Could you check a few things on this model? Use its own coordinates, in mm. A direction names the side the tool comes from. Round coordinates to 2 decimals unless told otherwise and drop trailing zeros. Loops run counter-clockwise (first coordinate to the right, second up) from the corner with the lowest first, then second, coordinate; pieces in that order, holes last. Notation, with made-up numbers: (15, 14.5) -> (31, 14.5) arc R22 ccw to (31, 52.5) -> close; hole circle Ø2 at (78.25, 31). An arc over 180 degrees is marked (long way). Write each question's results on one line, items separated by ' | '. Start each with the question number.
1) Imagine slicing it at B-B, the plane x = 0. List the corners of the cut face in (y, z) for me.
2) We'd pull the mould along X, two halves only. Please class faces 4 (the cylindrical face through (9.886, 0.74, 10.078)), 5 (the cylindrical face through (-0.108, 2.486, 0.488)), 6 (the flat face through (0, 0, 0)): pulls with the +X half, pulls with the -X half, needs draft (parallel to the pull), parting line crosses it, or undercut.
3) Imagine slicing it at C-C, the plane z = 2.5. List the corners of the cut face in (x, y) for me.
4) If I drill on probe 1 along Y at (x, z) = (9.5, -1.75); probe 2 along X at (y, z) = (1.2, -4); probe 3 along Y at (x, z) = (-4, 11.5), over which ranges is the centre line in solid material (lowest first)?
5) For P1, Ø1.3, axis at y = 3, z = 12.5, coming from the -X side; P2, Ø1.3, axis at y = 3, z = -13.5, coming from the +X side; P3, Ø1, axis at y = 4.5, z = -3, coming from the +X side; P4, Ø0.8, axis at x = 0, z = 0, coming from the +Y side, each with a flat end and sliding along its axis, tell me the tip position at first contact or that it passes through.
6) Imagine slicing it at A-A, the plane y = 2.95. List the corners of the cut face in (x, z) for me, plus the area to 3 significant figures.
7) Which directions (+Z, -Z, +X, -X, +Y, -Y) give clear straight access to the entire face, cutting with the end or side of a thin tool? Please do faces 1 (the flat face through (-13, 3, -1.25)), 2 (the flat face through (2, 0.5, 0)), 3 (the flat face through (1.25, 3, -13)).
8) Imagine slicing it at D-D, the plane z = -3. List the corners of the cut face in (x, y) for me.
from build123d import *

# Parameters (mm, degrees)
SKETCH1_W             = 1.2
SKETCH1_H             = 2.5
BOSS_EXTRUDE1_DEPTH   = 5.5
SKETCH1_W_2           = 2.5
SKETCH1_H_2           = 1.2
BOSS_EXTRUDE1_2_DEPTH = 5.5
BOSS_EXTRUDE1_3_DEPTH = 5.5
BOSS_EXTRUDE1_4_DEPTH = 5.5
SKETCH1_4_W           = 2.5
SKETCH1_4_H           = 2.5
BOSS_EXTRUDE2_DEPTH   = 0.5
BOSS_EXTRUDE3_DEPTH   = 1.5
SKETCH2_R             = 0.5
BOSS_EXTRUDE4_DEPTH   = 3
FILLET1_R             = 1


with BuildPart() as part:
    # Sketch1 → Boss-Extrude1 (new body)
    with BuildSketch(Plane(origin=(0, 0, 0), x_dir=(1, 0, 0), z_dir=(0, 1, 0))):
        with Locations((-13, 0)):
            Rectangle(SKETCH1_W, SKETCH1_H)
    extrude(amount=BOSS_EXTRUDE1_DEPTH)



with BuildPart() as body_2:
    # Sketch1 → Boss-Extrude1 2 (new body)
    with BuildSketch(Plane(origin=(0, 0, 0), x_dir=(1, 0, 0), z_dir=(0, 1, 0))):
        with Locations((0, 13)):
            Rectangle(SKETCH1_W_2, SKETCH1_H_2)
    extrude(amount=BOSS_EXTRUDE1_2_DEPTH)


with BuildPart() as body_3:
    # Sketch1 → Boss-Extrude1 3 (new body)
    with BuildSketch(Plane(origin=(0, 0, 0), x_dir=(1, 0, 0), z_dir=(0, 1, 0))):
        with Locations((13, 0)):
            Rectangle(SKETCH1_W, SKETCH1_H)
    extrude(amount=BOSS_EXTRUDE1_3_DEPTH)


with BuildPart() as body_4:
    # Sketch1 → Boss-Extrude1 4 (new body)
    with BuildSketch(Plane(origin=(0, 0, 0), x_dir=(1, 0, 0), z_dir=(0, 1, 0))):
        with Locations((0, -13)):
            Rectangle(SKETCH1_W_2, SKETCH1_H_2)
    extrude(amount=BOSS_EXTRUDE1_4_DEPTH)


with BuildPart() as body_5:
    # Sketch1<4> → Boss-Extrude2 (new body)
    with BuildSketch(Plane(origin=(0, 0, 0), x_dir=(1, 0, 0), z_dir=(0, 1, 0))):
        with BuildLine():
            ThreePointArc((-1.25, 11.934718262), (-8.485281374, 8.485281374), (-11.934718262, 1.25))
            Line((-11.934718262, 1.25), (-1.25, 1.25))
            Line((-1.25, 1.25), (-1.25, 11.934718262))
        make_face()
        with BuildLine():
            Line((1.25, 11.934718262), (1.25, 1.25))
            Line((1.25, 1.25), (11.934718262, 1.25))
            ThreePointArc((11.934718262, 1.25), (8.485281374, 8.485281374), (1.25, 11.934718262))
        make_face()
        with BuildLine():
            Line((-1.25, 11.934718262), (-1.25, 1.25))
            Line((-1.25, 1.25), (1.25, 1.25))
            Line((1.25, 1.25), (1.25, 11.934718262))
            ThreePointArc((1.25, 11.934718262), (0, 12), (-1.25, 11.934718262))
        make_face()
        with BuildLine():
            ThreePointArc((-11.934718262, 1.25), (-12, 0), (-11.934718262, -1.25))
            Line((-11.934718262, -1.25), (-1.25, -1.25))
            Line((-1.25, -1.25), (-1.25, 1.25))
            Line((-1.25, 1.25), (-11.934718262, 1.25))
        make_face()
        Rectangle(SKETCH1_4_W, SKETCH1_4_H)
        with BuildLine():
            Line((1.25, 1.25), (1.25, -1.25))
            Line((1.25, -1.25), (11.934718262, -1.25))
            ThreePointArc((11.934718262, -1.25), (11.983668452, -0.625851761), (12, 0))
            ThreePointArc((12, 0), (11.983668452, 0.625851761), (11.934718262, 1.25))
            Line((11.934718262, 1.25), (1.25, 1.25))
        make_face()
        with BuildLine():
            Line((11.934718262, -1.25), (1.25, -1.25))
            Line((1.25, -1.25), (1.25, -11.934718262))
            ThreePointArc((1.25, -11.934718262), (8.485281374, -8.485281374), (11.934718262, -1.25))
        make_face()
        with BuildLine():
            Line((-1.25, -1.25), (-11.934718262, -1.25))
            ThreePointArc((-11.934718262, -1.25), (-8.485281374, -8.485281374), (-1.25, -11.934718262))
            Line((-1.25, -11.934718262), (-1.25, -1.25))
        make_face()
        with BuildLine():
            Line((1.25, -1.25), (-1.25, -1.25))
            Line((-1.25, -1.25), (-1.25, -11.934718262))
            ThreePointArc((-1.25, -11.934718262), (0, -12), (1.25, -11.934718262))
            Line((1.25, -11.934718262), (1.25, -1.25))
        make_face()
    extrude(amount=BOSS_EXTRUDE2_DEPTH)


with BuildPart() as part_1:
    add(part.part)

    add(body_2.part)  # Boss-Extrude3 merges body 2

    add(body_3.part)  # Boss-Extrude3 merges body 3

    add(body_4.part)  # Boss-Extrude3 merges body 4

    add(body_5.part)  # Boss-Extrude3 merges body 5
    # Sketch1<5> → Boss-Extrude3 (add)
    with BuildSketch(Plane(origin=(0, 0, 0), x_dir=(1, 0, 0), z_dir=(0, 1, 0))):
        with BuildLine():
            ThreePointArc((-1.25, 13.6), (-9.982768748, 9.982768748), (-13.6, 1.25))
            Line((-13.6, 1.25), (-12.4, 1.25))
            Line((-12.4, 1.25), (-11.934718262, 1.25))
            ThreePointArc((-11.934718262, 1.25), (-8.485281374, 8.485281374), (-1.25, 11.934718262))
            Line((-1.25, 11.934718262), (-1.25, 12.4))
            Line((-1.25, 12.4), (-1.25, 13.6))
        make_face()
        with BuildLine():
            ThreePointArc((13.6, 1.25), (9.982768748, 9.982768748), (1.25, 13.6))
            Line((1.25, 13.6), (1.25, 12.4))
            Line((1.25, 12.4), (1.25, 11.934718262))
            ThreePointArc((1.25, 11.934718262), (8.485281374, 8.485281374), (11.934718262, 1.25))
            Line((11.934718262, 1.25), (12.4, 1.25))
            Line((12.4, 1.25), (13.6, 1.25))
        make_face()
        with BuildLine():
            Line((1.25, 12.4), (-1.25, 12.4))
            Line((-1.25, 12.4), (-1.25, 11.934718262))
            ThreePointArc((-1.25, 11.934718262), (0, 12), (1.25, 11.934718262))
            Line((1.25, 11.934718262), (1.25, 12.4))
        make_face()
        with BuildLine():
            Line((1.25, -12.4), (1.25, -13.6))
            ThreePointArc((1.25, -13.6), (9.982768748, -9.982768748), (13.6, -1.25))
            Line((13.6, -1.25), (12.4, -1.25))
            Line((12.4, -1.25), (11.934718262, -1.25))
            ThreePointArc((11.934718262, -1.25), (8.485281374, -8.485281374), (1.25, -11.934718262))
            Line((1.25, -11.934718262), (1.25, -12.4))
        make_face()
        with BuildLine():
            Line((11.934718262, -1.25), (12.4, -1.25))
            Line((12.4, -1.25), (12.4, 1.25))
            Line((12.4, 1.25), (11.934718262, 1.25))
            ThreePointArc((11.934718262, 1.25), (11.983668452, 0.625851761), (12, 0))
            ThreePointArc((12, 0), (11.983668452, -0.625851761), (11.934718262, -1.25))
        make_face()
        with BuildLine():
            Line((-12.4, -1.25), (-13.6, -1.25))
            ThreePointArc((-13.6, -1.25), (-9.982768748, -9.982768748), (-1.25, -13.6))
            Line((-1.25, -13.6), (-1.25, -12.4))
            Line((-1.25, -12.4), (-1.25, -11.934718262))
            ThreePointArc((-1.25, -11.934718262), (-8.485281374, -8.485281374), (-11.934718262, -1.25))
            Line((-11.934718262, -1.25), (-12.4, -1.25))
        make_face()
        with BuildLine():
            Line((-12.4, 1.25), (-12.4, -1.25))
            Line((-12.4, -1.25), (-11.934718262, -1.25))
            ThreePointArc((-11.934718262, -1.25), (-12, 0), (-11.934718262, 1.25))
            Line((-11.934718262, 1.25), (-12.4, 1.25))
        make_face()
        with BuildLine():
            Line((-1.25, -11.934718262), (-1.25, -12.4))
            Line((-1.25, -12.4), (1.25, -12.4))
            Line((1.25, -12.4), (1.25, -11.934718262))
            ThreePointArc((1.25, -11.934718262), (0, -12), (-1.25, -11.934718262))
        make_face()
    extrude(amount=BOSS_EXTRUDE3_DEPTH)

    # Sketch2 → Boss-Extrude4 (add)
    with BuildSketch(Plane(origin=(0, 0.5, 0), x_dir=(1, 0, 0), z_dir=(0, 1, 0))):
        Circle(SKETCH2_R)
    extrude(amount=BOSS_EXTRUDE4_DEPTH)

    # Fillet1
    fillet1_edges = [part_1.edges().sort_by_distance(p)[0] for p in [
        (-0.5, 0.5, 0),
    ]]
    fillet(fillet1_edges, radius=FILLET1_R)


solid = part_1.part
Checked values:
1) outline: (0, -13.6) -> (5.5, -13.6) -> (5.5, -12.4) -> (1.5, -12.4) -> (1.5, -12) -> (0.5, -12) -> (0.5, -1.5) arc R1 cw to (1.5, -0.5) -> (3.5, -0.5) -> (3.5, 0.5) -> (1.5, 0.5) arc R1 cw to (0.5, 1.5) -> (0.5, 12) -> (1.5, 12) -> (1.5, 12.4) -> (5.5, 12.4) -> (5.5, 13.6) -> (0, 13.6) -> close
2) face 4: pulls with the +X half | face 5: undercut | face 6: needs draft
3) outline: (-13.54, 0) -> (13.54, 0) -> (13.54, 1.5) -> (11.74, 1.5) -> (11.74, 0.5) -> (-11.74, 0.5) -> (-11.74, 1.5) -> (-13.54, 1.5) -> close
4) probe 1: 0 to 0.5 | probe 2: -13.29 to -11.31, 11.31 to 13.29 | probe 3: 0 to 1.5
5) P1: x = -1.25 | P2: x = 1.25 | P3: through | P4: y = 3.5
6) outline: (-13.6, -1.25) -> (-12.4, -1.25) -> (-12.4, 1.25) -> (-13.6, 1.25) -> close; (-1.25, -13.6) -> (1.25, -13.6) -> (1.25, -12.4) -> (-1.25, -12.4) -> close; (-1.25, 12.4) -> (1.25, 12.4) -> (1.25, 13.6) -> (-1.25, 13.6) -> close; circle Ø1 at (0, 0); (12.4, -1.25) -> (13.6, -1.25) -> (13.6, 1.25) -> (12.4, 1.25) -> close | area: 12.8 mm^2
7) face 1: -Z, +X, -X, +Y | face 2: +Y | face 3: +Z, -Z, +X, +Y
8) outline: (-13.48, 0) -> (13.48, 0) -> (13.48, 1.5) -> (11.62, 1.5) -> (11.62, 0.5) -> (-11.62, 0.5) -> (-11.62, 1.5) -> (-13.48, 1.5) -> close
